Can you work these out from the drawing? Everything is in mm from the part's minimum corner. A direction names the side the tool comes from. Round coordinates to 2 decimals unless told otherwise and drop trailing zeros. Loops run counter-clockwise (first coordinate to the right, second up) from the corner with the lowest first, then second, coordinate; pieces in that order, holes last. Notation, with made-up numbers: (7.25, 53.25) -> (25.25, 53.25) arc R15 cw to (25.25, 76.25) -> close; hole circle Ø3 at (47, -28). An arc over 180 degrees is marked (long way). One line per item, written item: value.
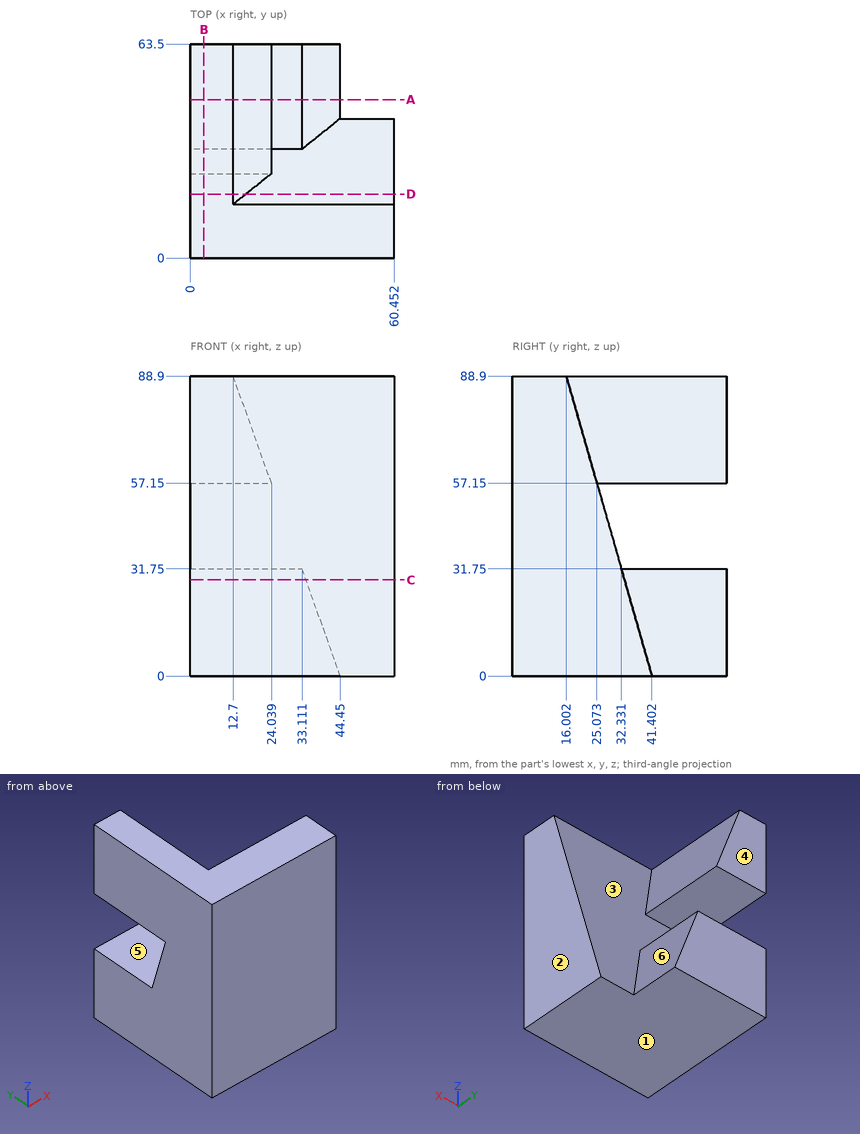
(1) Please list where these lines run through material, in increasing order: L1, parallel to Z at x = 9.5, y = 58; L2, parallel to Y at x = 35.5, z = 34.5 (1 decimal); L3, parallel to Y at x = 57, z = 12.5.
Results below:
L1: z = 0 to 31.75, 57.15 to 88.9
L2: y = 0 to 31.5
L3: y = 0 to 37.83
(2) We'd pull the mould along Z, two halves only. Please class the marked faces 1, 2 and 3: +Z half, -Z half, draft (parallel to the pull), parting line (faces both ways), or undercut.
Results below:
face 1: -Z half
face 2: draft
face 3: undercut
(3) Imagine slicing it at A-A on y = 47. Write out the boundary of the cut face in (x, z), then the cut area to 3 significant figures.
Results below:
outline: (0, 0) -> (44.45, 0) -> (33.11, 31.75) -> (0, 31.75) -> close; (0, 57.15) -> (24.04, 57.15) -> (12.7, 88.9) -> (0, 88.9) -> close
area: 1,810 mm²
(4) Imagine slicing it at C-C on z = 28.5. Write out the boundary of the cut face in (x, y).
Results below:
outline: (0, 0) -> (60.45, 0) -> (60.45, 33.26) -> (34.27, 33.26) -> (34.27, 63.5) -> (0, 63.5) -> close
(5) On a 3-axis mill with a long thin cutter (end or side, diameter ignored), from which of +Z, -Z, +X, -X, +Y, -Y can I reach the whole of each face in a straight line? I mean the marked faces 4, 5 and 6. Say none if no direction works.
Results below:
face 4: +Z, -Z, +X, -X, +Y
face 5: +X, -X, +Y
face 6: +Z, +X, +Y
(6) Imagine slicing it at B-B on x = 4. Write out the boundary of the cut face in (y, z), then the cut area to 3 significant figures.
Results below:
outline: (0, 0) -> (63.5, 0) -> (63.5, 31.75) -> (32.33, 31.75) -> (25.07, 57.15) -> (63.5, 57.15) -> (63.5, 88.9) -> (0, 88.9) -> close
area: 4,760 mm²
(7) Imagine slicing it at D-D on y = 19. Write out the boundary of the cut face in (x, z).
Results below:
outline: (0, 0) -> (60.45, 0) -> (60.45, 78.41) -> (16.45, 78.41) -> (12.7, 88.9) -> (0, 88.9) -> close
